Here's how the part is built. I have some questions about the finished solid (model axes, mm). A direction names the side the tool comes from. Coordinates: 2 decimals unless noted, no trailing zeros. Loops run counter-clockwise (first coordinate to the right, second up) from the corner with the lowest first, then second, coordinate; pieces in that order, holes last. Notation, with made-up numbers: (-28, 36) -> (25, 36) arc R15 ccw to (25, 44) -> close; hole circle Ø4 at (1, 59.25). An arc over 180 degrees is marked (long way). Answer as a JSON object with one key per item and string values. Group by question number.
Q1. I need wall thicknesses on line 1 (Z direction, x = 15, y = 35.75); line 2 (Y direction, x = -4.75, z = 15); line 3 (X direction, y = 28.5, z = 11.25). Which ranges of each line are inside material? Lowest first, please.
Q2. I want a section at D-D on x = -3. Write out the boundary of the cut face in (y, z), then the cut area to 3 significant figures.
Q3. On a 3-axis mill with a long thin cutter (end or side, diameter ignored), from which of +Z, -Z, +X, -X, +Y, -Y can I reach the whole of each face in a straight line? I mean faces 5 (the flat face through (-10, 20.3, 14.8)), 6 (the flat face through (0, 11, 11)). Say none if no direction works.
Q4. I want a section at C-C on y = 15. Write out the boundary of the cut face in (x, z), then the cut area to 3 significant figures.
Q5. I want a section at A-A on x = 15. Write out the boundary of the cut face in (y, z).
Q6. I want a section at B-B on z = 15. Write out the boundary of the cut face in (x, y).
Q7. I'm going to push flat-ended pins straight in: pin 1 (5 mm diameter, centred on x = 7, z = 10, fed in from -Y); pin 2 (13 mm diameter, centred on y = 15, z = 15, fed in from +X); pin 3 (12 mm diameter, centred on x = 1.5, y = 13, fed in from +Z). Where does each tip first touch, or does it pass through?
Q8. Thinking about a two-plate mould opening in Y: for faces 1 (the flat face through (30, 35, 15)), 2 (the flat face through (-5, 0, 15)), 3 (the flat face through (10, 40, 18)), 4 (the cylindrical face through (-4.93, 10.12, 16.08)), which applies, released by +Y, released by -Y, zero draft, split by the parting line, or undercut?
```python
from build123d import *

# Parameters (mm, degrees)
EXTRUDE_THIN1_DEPTH     = 30
SKETCH2_R               = 5
CUT_EXTRUDE1_DEPTH      = 31
CUT_EXTRUDE1_DEPTH_BACK = 11
SKETCH3_R               = 5
CUT_EXTRUDE2_DEPTH      = 11


with BuildPart() as part:
    # Sketch1 → Extrude-Thin1 (new body)
    with BuildSketch(Plane.XY):
        Polygon((0, 0), (0, 30), (30, 30), (30, 40), (-10, 40), (-10, 0), align=None)
    extrude(amount=EXTRUDE_THIN1_DEPTH)

    # Sketch2 → Cut-Extrude1 (cut, two sides)
    with BuildSketch(Plane(origin=(0, 30, 0), x_dir=(-1, 0, 0), z_dir=(0, -1, 0))) as cut_extrude1_sk:
        with Locations((-15, -15)):
            Circle(SKETCH2_R)
    extrude(amount=CUT_EXTRUDE1_DEPTH, mode=Mode.SUBTRACT)
    extrude(cut_extrude1_sk.sketch, amount=-CUT_EXTRUDE1_DEPTH_BACK, mode=Mode.SUBTRACT)

    # Sketch3 → Cut-Extrude2 (cut, through all)
    with BuildSketch(Plane(origin=(0, 0, 0), x_dir=(0, 0, -1), z_dir=(1, 0, 0))):
        with Locations((-15, 15)):
            Circle(SKETCH3_R)
    extrude(amount=-CUT_EXTRUDE2_DEPTH, mode=Mode.SUBTRACT)


solid = part.part
```
Result set:
{
 "1": {"line 1": "z = 0 to 10, 20 to 30", "line 2": "y = 0 to 10, 20 to 40", "line 3": "x = -10 to 0"},
 "2": {"outline": "(0, 0) -> (40, 0) -> (40, 30) -> (0, 30) -> close; hole circle Ø10 at (15, 15)", "area": "1,120 mm²"},
 "3": {"face 5": "+Z, -Z, -X, +Y, -Y", "face 6": "+Z, -Z, +X, -Y"},
 "4": {"outline": "(-10, 0) -> (0, 0) -> (0, 10) -> (-10, 10) -> close; (-10, 20) -> (0, 20) -> (0, 30) -> (-10, 30) -> close", "area": "200 mm²"},
 "5": {"outline": "(30, 0) -> (40, 0) -> (40, 10) -> (30, 10) -> close; (30, 20) -> (40, 20) -> (40, 30) -> (30, 30) -> close"},
 "6": {"outline": "(-10, 0) -> (0, 0) -> (0, 10) -> (-10, 10) -> close; (-10, 20) -> (0, 20) -> (0, 30) -> (10, 30) -> (10, 40) -> (-10, 40) -> close; (20, 30) -> (30, 30) -> (30, 40) -> (20, 40) -> close"},
 "7": {"pin 1": "stops at y = 30", "pin 2": "stops at x = 0", "pin 3": "stops at z = 30"},
 "8": {"face 1": "zero draft", "face 2": "released by -Y", "face 3": "released by +Y", "face 4": "undercut"}
}
